Can you work these out from the model? Positions are in its coordinate system, mm. Give positions to 0.01 mm unless a question says otherwise; leave off trailing zeros. Order: outer loops, then holes, each group sorted by start corner. A loop starts at its lowest first (then second) coordinate and runs counter-clockwise, first axis right, second up. Notation, with made-up numbers: (-28.5, 53) - (4.5, 53) arc R18 ccw to (4.5, 72) - close; hole circle Ø7 at (26, 11.25). An arc over 180 degrees is marked (long way). Return JSON: item names as keys, results as strings.
```python
from build123d import *

# Parameters (mm, degrees)
PAD_DEPTH       = 3
SKETCH001_R     = 2.6
POCKET_DEPTH    = 39.421276
SKETCH002_W     = 42
SKETCH002_H     = 14
PAD001_DEPTH    = 5
SKETCH003_W     = 25
SKETCH003_H     = 24
PAD002_DEPTH    = 3
PAD003_DEPTH    = 5.25
PAD004_DEPTH    = 3
SKETCH006_R     = 2.6
POCKET001_DEPTH = 39.421276
SKETCH007_W     = 10.046043
SKETCH007_H     = 6.845245
POCKET002_DEPTH = 24.040304
POCKET003_DEPTH = 24.001
POCKET004_DEPTH = 57.585803
SKETCH009_R     = 1.5
POCKET005_DEPTH = 7.276792
FILLET_R        = 1


with BuildPart() as part:
    # Sketch → Pad (new body)
    with BuildSketch(Plane.XY):
        Polygon((-111.071915, -107.875351), (-111.592859, -104.920928), (-86.972666, -100.579724), (-86.451721, -103.534147), (-21, -135), (21, -135), (21, -140), (-21, -140), align=None)
    extrude(amount=PAD_DEPTH)

    # Sketch001 (on Face7 of Pad) → Pocket (cut, through all)
    with BuildSketch(Plane.XZ.offset(140)):
        with Locations((-11.143028, 7)):
            Circle(SKETCH001_R)
        with Locations((11.143028, 7)):
            Circle(SKETCH001_R)
    extrude(amount=-POCKET_DEPTH, mode=Mode.SUBTRACT)

    # Sketch002 (on Face7 of Pad) → Pad001 (join)
    with BuildSketch(Plane.XZ.offset(140)):
        with Locations((0, 7)):
            Rectangle(SKETCH002_W, SKETCH002_H)
    extrude(amount=-PAD001_DEPTH)

    # Sketch003 (on Face3 of Pad001) → Pad002 (join)
    with BuildSketch(Plane(origin=(14.577599, -82.673672, 0), x_dir=(-0.984808, -0.173648, 0), z_dir=(-0.173648, 0.984808, 0))):
        with Locations((115.62, 12)):
            Rectangle(SKETCH003_W, SKETCH003_H)
    extrude(amount=-PAD002_DEPTH)

    # Sketch004 (on Face14 of Pad002) → Pad003 (join)
    with BuildSketch(Plane(origin=(-46.66687, -130.845768, 0), x_dir=(0.941887, -0.335929, 0), z_dir=(-0.335929, -0.941887, 0))):
        Polygon((27.29, 14), (-68.35, 24), (-68.35, 21), (27.29, 11), align=None)
    extrude(amount=-PAD003_DEPTH)

    # Sketch005 (on Face25 of Pad003) → Pad004 (join)
    with BuildSketch(Plane(origin=(1.641818, -0.585563, 16.671151), x_dir=(0.995191, 0.003438, -0.097888), z_dir=(0.097949, -0.034934, 0.994578))):
        Polygon((-88.519324, -102.708058), (-20.951239, -134.433376), (-22.737431, -139.436564), (-113.251967, -106.97329), (-113.372097, -106.249408), (-88.616976, -102.170205), align=None)
    extrude(amount=-PAD004_DEPTH)

    # Sketch006 (on Face36 of Pad004) → Pocket001 (cut, through all)
    with BuildSketch(Plane.XZ.offset(140)):
        with Locations((-16, 7)):
            Circle(SKETCH006_R)
        with Locations((16, 7)):
            Circle(SKETCH006_R)
    extrude(amount=-POCKET001_DEPTH, mode=Mode.SUBTRACT)

    # Sketch007 (on Face17 of Pocket001) → Pocket002 (cut, through all)
    with BuildSketch(Plane(origin=(0, 0, 0), x_dir=(1, 0, 0), z_dir=(0, 0, -1))):
        with Locations((-15.976978, 131.577378)):
            Rectangle(SKETCH007_W, SKETCH007_H)
    extrude(amount=-POCKET002_DEPTH, mode=Mode.SUBTRACT)

    # Sketch008 (on Face10 of Pocket002) → Pocket003 (cut, through all)
    with BuildSketch(Plane.XY.offset(24)):
        Polygon((-111.59565, -104.921097), (-104.281212, -103.631622), (-103.238319, -101.954292), (-111.59565, -102.358459), align=None)
    extrude(amount=-POCKET003_DEPTH, mode=Mode.SUBTRACT)

    # Sketch010 (on Face4 of Pocket003) → Pocket004 (cut, through all)
    with BuildSketch(Plane(origin=(14.577599, -82.673672, 0), x_dir=(-0.984808, -0.173648, 0), z_dir=(-0.173648, 0.984808, 0))):
        Polygon((127.009121, 24), (128.119995, 24), (128.119995, 20.625757), (128.829539, 20.625757), (128.829539, 24.40741), (126.853241, 24.40741), align=None)
    extrude(amount=-POCKET004_DEPTH, mode=Mode.SUBTRACT)

    # Sketch009 (on Face20 of Pocket003) → Pocket005 (cut, through all)
    with BuildSketch(Plane(origin=(15.098544, -85.628095, 0), x_dir=(0.984808, 0.173648, 0), z_dir=(0.173648, -0.984808, 0))):
        with Locations((-124, 17)):
            Circle(SKETCH009_R)
        with Locations((-108, 15)):
            Circle(SKETCH009_R)
        with Locations((-124, 7)):
            Circle(SKETCH009_R)
        with Locations((-108, 7)):
            Circle(SKETCH009_R)
    extrude(amount=-POCKET005_DEPTH, mode=Mode.SUBTRACT)

    # Fillet
    fillet_edges = [part.edges().sort_by_distance(p)[0] for p in [
        (21, -137.5, 14),
        (21, -137.5, 0),
    ]]
    fillet(fillet_edges, radius=FILLET_R)


solid = part.part
```
1. Suppose I cut it at D-D (x = -101). List the corners of the cut face in (y, z) for me, plus the area to 3 significant figures.
Checks:
{"outline": "(-111.47, 0) - (-103.05, 0) - (-103.05, 24) - (-106.1, 24) - (-106.1, 23.07) - (-111.47, 22.88) - (-111.47, 19.87) - (-106.1, 20.06) - (-106.1, 3) - (-111.47, 3) - close", "area": "105 mm^2"}
2. Thinking about a two-plate mould opening in X: for faces 1 (the face through (18.48, -137.54, 7.78)), 2 (the face through (-111.34, -106.38, 10.17)), 3 (the face through (-13.52, -137.54, 7.78)), 4 (the face through (5, -135, 7)), which applies, +X half, -X half, draft (parallel to the pull), parting line (faces both ways), or undercut?
Checks:
{"face 1": "undercut", "face 2": "-X half", "face 3": "undercut", "face 4": "draft"}
3. Suppose I cut it at B-B (z = 7). List the corners of the cut face in (x, y) for me, plus the area to 3 significant figures.
Checks:
{"outline": "(-111.6, -104.92) - (-111.08, -107.88) - (-108.49, -107.42) - (-109.02, -104.47) - close; (-106.06, -103.95) - (-105.54, -106.9) - (-92.74, -104.64) - (-93.26, -101.69) - close; (-90.3, -101.17) - (-89.78, -104.12) - (-86.45, -103.53) - (-86.98, -100.58) - close; (-21, -140) - (-18.6, -140) - (-18.6, -135) - (-21, -135) - close; (-13.4, -140) - (13.4, -140) - (13.4, -135) - (-13.4, -135) - close; (18.6, -140) - (21, -140) - (21, -135) - (18.6, -135) - close", "area": "215 mm^2"}
4. If I drill on L1, parallel to Z at x = -16, y = -138; L2, parallel to Z at x = -82.5, y = -105.5; L3, parallel to Y at x = -2, z = 13.5, over which ranges is the centre line in solid material (lowest first)? Write a range as [from, to].
Checks:
{"L1": "[0, 4.4], [9.6, 14]", "L2": "[0, 3], [18.26, 21.27]", "L3": "[-140, -135]"}
5. Suppose I cut it at C-C (y = -121). List the corners of the cut face in (x, z) for me.
Checks:
{"outline": "(-74.29, 16.9) - (-49.21, 14.43) - (-49.14, 17.44) - (-74.29, 19.92) - close; (-74.27, 0) - (-50.12, 0) - (-50.12, 3) - (-74.27, 3) - close"}
6. For pin 1 Ø5 at (x, y) = (-43.5, -127) entering from +Z; pin 2 Ø4 at (x, z) = (-40, 11) entering from +Y; pin 3 Ø0.6 at (x, y) = (-111.5, -106) entering from +Z; pin 4 Ø8 at (x, z) = (-30.5, 14.5) entering from -Y, each with a flat end and sliding along its axis, tell me the tip position at first contact or that it passes through.
Checks:
{"pin 1": "z = 16.94", "pin 2": "through", "pin 3": "z = 24", "pin 4": "y = -138.05"}
7. Suppose I cut it at A-A (x = 16). List the corners of the cut face in (y, z) for me, plus the area to 3 significant figures.
Checks:
{"outline": "(-140, 0) - (-135, 0) - (-135, 4.4) - (-140, 4.4) - close; (-140, 9.6) - (-135, 9.6) - (-135, 14) - (-140, 14) - close", "area": "44.0 mm^2"}
